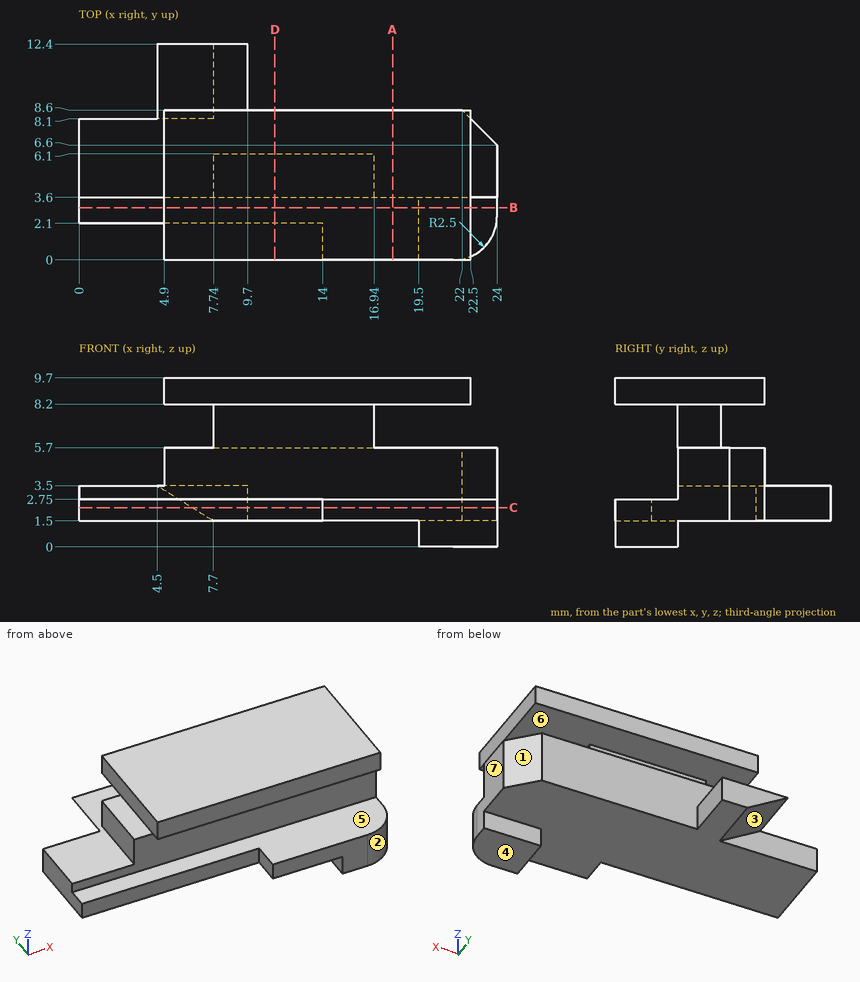
For this review, use the dimensioned drawing (mm, ordinates from the lowest corner) and the shaded views. A direction names the side the tool comes from. Give positions to 0.01 mm unless a question says otherwise; leave off trailing zeros. Order: outer loops, then holes, each group sorted by start corner. A loop starts at its lowest first (then second) coordinate and runs counter-clockwise, first axis right, second up. Notation, with made-up numbers: (-30, 51) - (26, 51) arc R22 ccw to (26, 89) - close; hole circle Ø3 at (-7.5, 84). An arc over 180 degrees is marked (long way). Use a Markdown table: item, result. Add a question column.
(1) Add section D-D on x = 11.25. Give the boundary of the cut face in (y, z), then the cut area to 3 significant figures.
(2) Wall thickness on probe 1 along Z at (x, y) = (19, 7.5); probe 2 along Z at (x, y) = (16, 0.5); probe 3 along Y at (x, z) = (14.75, 7): over which ranges is each line inside the solid? List them lowest first. Write a range as [from, to].
(3) Add section C-C on z = 2.25. Give the boundary of the cut face in (x, y), then the cut area to 3 significant figures.
(4) Machinability: for the marked faces 1, 2 and 3, which of the approach directions +Z, -Z, +X, -X, +Y, -Y give a long, thin tool a straight path to every point of the face, cutting with its end or side? Answer none if there is none.
(5) Add section B-B on y = 3. Give the boundary of the cut face in (x, z).
(6) Clearance check with flat-ended pins moving along their axes: P1, Ø0.6, axis at x = 3.5, z = 3, coming from the +Y side; P2, Ø1, axis at x = 18.5, z = 4.5, coming from the +Y side; P3, Ø1.6, axis at y = 2.5, z = 0.5, coming from the -X side. State where each tip first meets the part, or that it passes through.
(7) Add section A-A on x = 18. Give the boundary of the cut face in (y, z), then the cut area to 3 significant figures.
(8) Mouldability with a two-part tool opening along Z and no side actions: class the marked faces 4, 5, 6 and 7 as +Z half, -Z half, draft (parallel to the pull), parting line (faces both ways), or undercut.
Report:
| question | item | result |
|---|---|---|
| 1 | outline | (0, 8.2) - (3.6, 8.2) - (3.6, 2.75) - (2.1, 2.75) - (2.1, 1.5) - (8.6, 1.5) - (8.6, 5.7) - (6.1, 5.7) - (6.1, 8.2) - (8.6, 8.2) - (8.6, 9.7) - (0, 9.7) - close |
| 1 | area | 42.0 mm² |
| 2 | probe 1 | z = [1.5, 5.7], [8.2, 9.7] |
| 2 | probe 2 | z = [1.5, 2.75], [8.2, 9.7] |
| 2 | probe 3 | y = [3.6, 6.1] |
| 3 | outline | (0, 2.1) - (14, 2.1) - (14, 0) - (21.5, 0) arc R2.5 ccw to (24, 2.5) - (24, 6.6) - (22, 8.6) - (9.7, 8.6) - (9.7, 12.4) - (6.5, 12.4) - (6.5, 8.1) - (0, 8.1) - close |
| 3 | area | 183 mm² |
| 4 | face 1 | -Z, +X, +Y |
| 4 | face 2 | -Z, +X, -Y |
| 4 | face 3 | -Z, -X, +Y |
| 5 | outline | (0, 1.5) - (19.5, 1.5) - (19.5, 0) - (24, 0) - (24, 2.75) - (0, 2.75) - close; (4.9, 8.2) - (22.5, 8.2) - (22.5, 9.7) - (4.9, 9.7) - close |
| 6 | P1 | stops at y = 8.1 |
| 6 | P2 | stops at y = 8.6 |
| 6 | P3 | stops at x = 19.5 |
| 7 | outline | (0, 1.5) - (8.6, 1.5) - (8.6, 5.7) - (3.6, 5.7) - (3.6, 2.75) - (0, 2.75) - close; (0, 8.2) - (8.6, 8.2) - (8.6, 9.7) - (0, 9.7) - close |
| 7 | area | 38.4 mm² |
| 8 | face 4 | -Z half |
| 8 | face 5 | undercut |
| 8 | face 6 | undercut |
| 8 | face 7 | draft |
